from build123d import *

# Parameters (mm, degrees)
SKETCH1_R               = 16
BOSS_EXTRUDE1_DEPTH     = 3
SKETCH2_R               = 8
BOSS_EXTRUDE2_DEPTH     = 10
CUT_EXTRUDE1_REACH      = 28.096
SKETCH3_R               = 4
CUT_EXTRUDE2_REACH      = 26.739
SKETCH4_R               = 2.25
CUT_EXTRUDE3_REACH      = 28.096
CUT_EXTRUDE3_END_RADIUS = 8
SKETCH5_R               = 2


with BuildPart() as part:
    # Sketch1 → Boss-Extrude1 (new body)
    with BuildSketch(Plane(origin=(0, 0, 0), x_dir=(1, 0, 0), z_dir=(0, 1, 0))):
        with Locations(Location((0, 0, 0), (0, 0, 270))):
            Circle(SKETCH1_R)
    extrude(amount=BOSS_EXTRUDE1_DEPTH)

    # Sketch2 → Boss-Extrude2 (add)
    with BuildSketch(Plane(origin=(0, 3, 0), x_dir=(1, 0, 0), z_dir=(0, 1, 0))):
        with Locations(Location((0, 0, 0), (0, 0, 270))):
            Circle(SKETCH2_R)
    extrude(amount=BOSS_EXTRUDE2_DEPTH)

    # Sketch3 → Cut-Extrude1 (cut, up to next)
    with BuildSketch(Plane(origin=(0, 13, 0), x_dir=(1, 0, 0), z_dir=(0, 1, 0)), mode=Mode.PRIVATE) as cut_extrude1_sk1:
        with Locations(Location((0, 0, 0), (0, 0, 270))):
            Circle(SKETCH3_R)
    cut_extrude1_tool1 = extrude(cut_extrude1_sk1.sketch, amount=-CUT_EXTRUDE1_REACH, mode=Mode.PRIVATE) & part.part
    add(cut_extrude1_tool1.solids().sort_by_distance((0, 13, 0))[0], mode=Mode.SUBTRACT)

    # Sketch4 → Cut-Extrude2 (cut, up to next)
    with BuildSketch(Plane(origin=(0, 3, 0), x_dir=(1, 0, 0), z_dir=(0, 1, 0)), mode=Mode.PRIVATE) as cut_extrude2_sk1:
        with Locations(Location((0, 12, 0), (0, 0, 270))):
            Circle(SKETCH4_R)
    cut_extrude2_tool1 = extrude(cut_extrude2_sk1.sketch, amount=-CUT_EXTRUDE2_REACH, mode=Mode.PRIVATE) & part.part
    # Sketch4 → Cut-Extrude2 (cut, up to next)
    with BuildSketch(Plane(origin=(0, 3, 0), x_dir=(1, 0, 0), z_dir=(0, 1, 0)), mode=Mode.PRIVATE) as cut_extrude2_sk2:
        with Locations(Location((12, 0, 0), (0, 0, 270))):
            Circle(SKETCH4_R)
    cut_extrude2_tool2 = extrude(cut_extrude2_sk2.sketch, amount=-CUT_EXTRUDE2_REACH, mode=Mode.PRIVATE) & part.part
    # Sketch4 → Cut-Extrude2 (cut, up to next)
    with BuildSketch(Plane(origin=(0, 3, 0), x_dir=(1, 0, 0), z_dir=(0, 1, 0)), mode=Mode.PRIVATE) as cut_extrude2_sk3:
        with Locations(Location((0, -12, 0), (0, 0, 270))):
            Circle(SKETCH4_R)
    cut_extrude2_tool3 = extrude(cut_extrude2_sk3.sketch, amount=-CUT_EXTRUDE2_REACH, mode=Mode.PRIVATE) & part.part
    # Sketch4 → Cut-Extrude2 (cut, up to next)
    with BuildSketch(Plane(origin=(0, 3, 0), x_dir=(1, 0, 0), z_dir=(0, 1, 0)), mode=Mode.PRIVATE) as cut_extrude2_sk4:
        with Locations(Location((-12, 0, 0), (0, 0, 270))):
            Circle(SKETCH4_R)
    cut_extrude2_tool4 = extrude(cut_extrude2_sk4.sketch, amount=-CUT_EXTRUDE2_REACH, mode=Mode.PRIVATE) & part.part
    add(cut_extrude2_tool1.solids().sort_by_distance((0, 3, -12))[0], mode=Mode.SUBTRACT)
    add(cut_extrude2_tool2.solids().sort_by_distance((12, 3, 0))[0], mode=Mode.SUBTRACT)
    add(cut_extrude2_tool3.solids().sort_by_distance((0, 3, 12))[0], mode=Mode.SUBTRACT)
    add(cut_extrude2_tool4.solids().sort_by_distance((-12, 3, 0))[0], mode=Mode.SUBTRACT)

    # Cut-Extrude3: up to this cylinder (the profile starts inside it)
    cut_extrude3_end = Plane(origin=(0, 8, 0), z_dir=(0, -1, 0)) * Cylinder(CUT_EXTRUDE3_END_RADIUS, 73.192, mode=Mode.PRIVATE)
    # Sketch5 → Cut-Extrude3 (cut, up to the surface)
    with BuildSketch(Plane.XY, mode=Mode.PRIVATE) as cut_extrude3_sk1:
        with Locations((0, 8)):
            Circle(SKETCH5_R)
    cut_extrude3_tool1 = extrude(cut_extrude3_sk1.sketch, amount=-CUT_EXTRUDE3_REACH, mode=Mode.PRIVATE) & cut_extrude3_end
    add(cut_extrude3_tool1.solids().sort_by_distance((0, 8, 0))[0], mode=Mode.SUBTRACT)


solid = part.part
Read the model definition and answer for the solid it produces. Units are mm, in the model's axes. A direction names the side the tool comes from. Round coordinates to 2 decimals unless told otherwise and drop trailing zeros. Write each loop counter-clockwise with the first axis right and the second up, starting at its lowest first coordinate (ties: lowest second). Pieces come first, ordered by that corner, then holes. Notation, with made-up numbers: M 73,4.25 L 108,4.25 A31 ccw 108,34.25 Z; hole C 60.25,0 d8. An arc over 180 degrees is marked long. Use a Markdown table: item, result.
1) The part is cut by section B-B (z = 0). Write down the section's boundary in (x, y), plus the area to 3 significant figures.
Answers follow:
| item | result |
|---|---|
| outline | M -16,0 L -14.25,0 L -14.25,3 L -16,3 Z; M -9.75,0 L -4,0 L -4,13 L -8,13 L -8,3 L -9.75,3 Z; M 4,0 L 9.75,0 L 9.75,3 L 8,3 L 8,13 L 4,13 Z; M 14.25,0 L 16,0 L 16,3 L 14.25,3 Z |
| area | 125 mm2 |
2) Flat-ended cylindrical pins translate along their axes: pin 1 (12 mm diameter, centred on x = -12, z = 7, fed in from -Y); pin 2 (6 mm diameter, centred on x = 4.5, y = 7.5, fed in from -Z); pin 3 (4 mm diameter, centred on x = -9.5, y = 2, fed in from -Z); pin 4 (6 mm diameter, centred on x = -6.5, z = -11, fed in from +Y). Find the tip coordinate at first contact, or state that the pin passes through.
Answers follow:
| item | result |
|---|---|
| pin 1 | stops at y = 0 |
| pin 2 | stops at z = -7.84 |
| pin 3 | stops at z = -14.13 |
| pin 4 | stops at y = 3 |
3) The part is cut by section A-A (x = 0). Write down the section's boundary in (y, z).
Answers follow:
| item | result |
|---|---|
| outline | M 0,-16 L 3,-16 L 3,-14.25 L 0,-14.25 Z; M 0,-9.75 L 3,-9.75 L 3,-8 L 6,-8 L 6,-4 L 0,-4 Z; M 0,4 L 13,4 L 13,8 L 3,8 L 3,9.75 L 0,9.75 Z; M 0,14.25 L 3,14.25 L 3,16 L 0,16 Z; M 10,-8 L 13,-8 L 13,-4 L 10,-4 Z |
4) Straight lines are drawn through the part: line 1 along X through (y, z) = (1.7, 0); line 2 along X through (y, z) = (5, 0). For each, find the intervals that lie inside material, in ascending order. Write a range as [from, to].
Answers follow:
| item | result |
|---|---|
| line 1 | x = [-16, -14.25], [-9.75, -4], [4, 9.75], [14.25, 16] |
| line 2 | x = [-8, -4], [4, 8] |
5) For a pull along X with two mould halves and no side action, classify faces 4 (the cylindrical face through (-1.532, 6.591, 3.695)), 5 (the cylindrical face through (-3.06, 7.93, 7.39)), 6 (the flat face through (-3, 0, 3)), 7 (the cylindrical face through (0.099, 1.521, 9.752)) as pulls with the +X half, pulls with the -X half, needs draft (parallel to the pull), parting line crosses it, or undercut.
Answers follow:
| item | result |
|---|---|
| face 4 | undercut |
| face 5 | parting line crosses it |
| face 6 | needs draft |
| face 7 | undercut |
6) A tool of negligible diameter and unlimited length cuts with its end or side. For faces 1 (the flat face through (3.8, 3, -7.3)), 2 (the cylindrical face through (0.923, 6.226, -5.7)), 3 (the flat face through (-2, 13, -4)), from which of +Z, -Z, +X, -X, +Y, -Y can it reach the whole face along a straight path? Write none if from no direction.
Answers follow:
| item | result |
|---|---|
| face 1 | +Y |
| face 2 | -Z |
| face 3 | +Z, -Z, +X, -X, +Y |
7) The part is cut by section C-C (y = 2.25). Write down the section's boundary in (x, z).
Answers follow:
| item | result |
|---|---|
| outline | C 0,0 d32; hole C -12,0 d4.5; hole C 0,0 d8; hole C 0,-12 d4.5; hole C 0,12 d4.5; hole C 12,0 d4.5 |
8) The part is cut by section D-D (z = -12). Write down the section's boundary in (x, y), plus the area to 3 significant figures.
Answers follow:
| item | result |
|---|---|
| outline | M -10.58,0 L -2.25,0 L -2.25,3 L -10.58,3 Z; M 2.25,0 L 10.58,0 L 10.58,3 L 2.25,3 Z |
| area | 50.0 mm2 |
